For this review, take the finished solid that the model builds, in its own axes (mm). Face numbers are marked on the shaded views. A direction names the side the tool comes from. Round coordinates to 2 decimals unless told otherwise and drop trailing zeros. Loops run counter-clockwise (first coordinate to the right, second up) from the corner with the lowest first, then second, coordinate; pieces in that order, holes last. Notation, with made-up numbers: M 17,22.5 L 49,22.5 A28 ccw 49,43.5 Z; hole C 53.25,26 d6. An arc over 180 degrees is marked long. Write item = value, one per line. Start each with the question number.
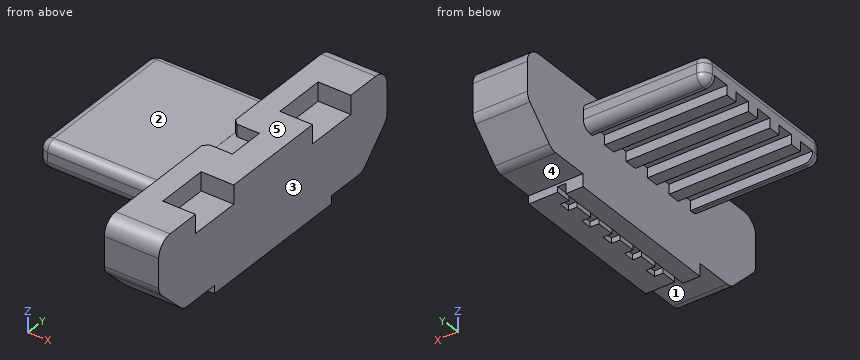
```python
from build123d import *

# Parameters (mm, degrees)
PAD009_DEPTH    = 1.8
PAD008_DEPTH    = 1.2
SKETCH018_W     = 0.214
SKETCH018_H     = 0.247
POCKET007_DEPTH = 0.119
SKETCH019_W     = 0.72
SKETCH019_H     = 1.16
POCKET008_DEPTH = 0.414
POCKET009_DEPTH = 0.27
PAD013_DEPTH    = 2.7
FILLET001_R     = 0.2


with BuildPart() as pad009:
    # Sketch017 → Pad009 (new body, symmetric)
    with BuildSketch(Plane.XZ):
        Polygon((1.529, 0), (1.529, 0.264), (1.708, 0.264), (1.708, 0.145), (2.358, 0.145), (2.358, 0), align=None)
    extrude(amount=PAD009_DEPTH, both=True)


with BuildPart() as part_back:
    # Sketch016 → Pad008 (new body)
    with BuildSketch(Plane(origin=(1.1499999635, -0.0083336435, -0.0078429583), x_dir=(0, 1, 0), z_dir=(1, 0, 0))):
        with BuildLine():
            Line((-3.1093336572, 2.1718425317), (3.1093336572, 2.1718425317))
            ThreePointArc((3.4533336572, 1.8278425317), (3.35257839, 2.0710872645), (3.1093336572, 2.1718425317))
            Line((3.4533336572, 1.8278425317), (3.4533336572, 1.1848425317))
            ThreePointArc((3.3757169542, 0.9974592347), (3.4331617333, 1.0834314222), (3.4533336572, 1.1848425317))
            Line((2.7923538598, 0.4140961402), (3.3757169542, 0.9974592347))
            ThreePointArc((2.588, 0.32945), (2.698595512, 0.3514488151), (2.7923538598, 0.4140961402))
            Line((1.77, 0.32945), (2.588, 0.32945))
            Line((1.77, 0.05045), (1.77, 0.32945))
            Line((1.77, 0.05045), (-1.77, 0.05045))
            Line((-1.77, 0.05045), (-1.77, 0.32945))
            Line((-1.77, 0.32945), (-2.588, 0.32945))
            ThreePointArc((-2.7923538598, 0.4140961402), (-2.698595512, 0.3514488151), (-2.588, 0.32945))
            Line((-3.3757169542, 0.9974592347), (-2.7923538598, 0.4140961402))
            ThreePointArc((-3.4533336572, 1.1848425317), (-3.4331617333, 1.0834314222), (-3.3757169542, 0.9974592347))
            Line((-3.4533336572, 1.8278425317), (-3.4533336572, 1.1848425317))
            ThreePointArc((-3.1093336572, 2.1718425317), (-3.35257839, 2.0710872645), (-3.4533336572, 1.8278425317))
        make_face()
    extrude(amount=PAD008_DEPTH)

    # Cut: cut Pad009
    add(pad009.part, mode=Mode.SUBTRACT)

    # Sketch018 (on Face19 of Cut) → Pocket007 (cut)
    with BuildSketch(Plane(origin=(0, 0, 0.145), x_dir=(1, 0, 0), z_dir=(0, 0, -1))):
        with Locations((1.792, -1.3005)):
            Rectangle(SKETCH018_W, SKETCH018_H)
        with Locations((1.792, -0.6435)):
            Rectangle(SKETCH018_W, SKETCH018_H)
        with Locations((1.792, 0)):
            Rectangle(SKETCH018_W, SKETCH018_H)
        with Locations((1.792, 0.6435)):
            Rectangle(SKETCH018_W, SKETCH018_H)
        with Locations((1.792, 1.3005)):
            Rectangle(SKETCH018_W, SKETCH018_H)
    extrude(amount=-POCKET007_DEPTH, mode=Mode.SUBTRACT)

    # Sketch019 (on Face2 of Pocket007) → Pocket008 (cut)
    with BuildSketch(Plane.XY.offset(2.1639995734)):
        with Locations((1.9899999635, -1.771)):
            Rectangle(SKETCH019_W, SKETCH019_H)
        with Locations((1.9899999635, 1.771)):
            Rectangle(SKETCH019_W, SKETCH019_H)
    extrude(amount=-POCKET008_DEPTH, mode=Mode.SUBTRACT)

    # Sketch020 (on Face2 of Pocket008) → Pocket009 (cut)
    with BuildSketch(Plane.XY.offset(2.1639995734)):
        Polygon((1.249, 0.41), (1.749, 0.41), (1.749, -0.41), (1.249, -0.41), (1.146, -0.513), (1.146, 0.513), align=None)
    extrude(amount=-POCKET009_DEPTH, mode=Mode.SUBTRACT)


with BuildPart() as inner:
    # Sketch029 → Pad013 (new body)
    with BuildSketch(Plane(origin=(-1.5500000108, 1.37e-08, -0.0050004214), x_dir=(0, 1, 0), z_dir=(1, 0, 0))):
        with BuildLine():
            Line((-1.75, 1.6999999949), (-1.75, 1.5000000051))
            ThreePointArc((-1.75, 1.5000000051), (-1.6914213581, 1.3585786456), (-1.55, 1.3))
            Line((-1.55, 1.3), (-1.486, 1.3))
            Line((-1.486, 1.3), (-1.486, 1.514))
            Line((-1.486, 1.514), (-1.115, 1.514))
            Line((-1.115, 1.514), (-1.115, 1.3))
            Line((-1.115, 1.3), (-0.837, 1.3))
            Line((-0.837, 1.3), (-0.837, 1.514))
            Line((-0.837, 1.514), (-0.466, 1.514))
            Line((-0.466, 1.514), (-0.466, 1.3))
            Line((-0.466, 1.3), (-0.188, 1.3))
            Line((-0.188, 1.3), (-0.188, 1.514))
            Line((-0.188, 1.514), (0.183, 1.514))
            Line((0.183, 1.514), (0.183, 1.3))
            Line((0.183, 1.3), (0.461, 1.3))
            Line((0.461, 1.3), (0.461, 1.514))
            Line((0.461, 1.514), (0.832, 1.514))
            Line((0.832, 1.514), (0.832, 1.3))
            Line((0.832, 1.3), (1.11, 1.3))
            Line((1.11, 1.3), (1.11, 1.514))
            Line((1.11, 1.514), (1.481, 1.514))
            Line((1.481, 1.514), (1.481, 1.3))
            Line((1.481, 1.3), (1.55, 1.3))
            ThreePointArc((1.55, 1.3), (1.6914213581, 1.3585786456), (1.75, 1.5000000051))
            Line((1.75, 1.6999999949), (1.75, 1.5000000051))
            ThreePointArc((1.75, 1.6999999949), (1.6914213581, 1.8414213544), (1.55, 1.9))
            Line((-1.55, 1.9), (1.55, 1.9))
            ThreePointArc((-1.55, 1.9), (-1.6914213581, 1.8414213544), (-1.75, 1.6999999949))
        make_face()
    extrude(amount=PAD013_DEPTH)

    # Fillet001
    fillet001_edges = [inner.edges().sort_by_distance(p)[0] for p in [
        (-1.55, -1.75, 1.595),
        (-1.55, -1.691421, 1.353578),
        (-1.55, 1.691421, 1.353578),
        (-1.55, 1.75, 1.595),
        (-1.55, 1.691421, 1.836421),
        (-1.55, 0, 1.895),
        (-1.55, -1.691421, 1.836421),
    ]]
    fillet(fillet001_edges, radius=FILLET001_R)

    # Fusion002: union Part-back
    add(part_back.part)


solid = inner.part
```
(1) Wall thickness on L1, parallel to Y at x = 2.15, z = 1.8 (3 decimals); L2, parallel to X at y = 0.5, z = 0.8; L3, parallel to Z at x = 1.75, y = -2.5: over which ranges is each line inside the solid? List them lowest first.
(2) Add section C-C on x = 0.4. Write out the cut boundary in (y, z) (3 decimals), and give its area (3 significant figures).
(3) Add section A-A on x = 2.15. Write out the cut boundary in (y, z) (3 decimals), and give its area (3 significant figures).
(4) Tool access review of the marked faces 1, 2, 3, 4 and 5: name each direction out of +Z, -Z, +X, -X, +Y, -Y from which nothing blocks a thin tool from reaching the whole face with its end or side.
(5) Add section B-B on y = 2. Write out the cut boundary in (x, z), and give its area (3 significant figures).
(6) For pin 1 Ø0.7 at (x, y) = (2, -2) entering from -Z (3 decimals), flat-tipped, find the tip position at first contact; note if it passes through.
Answer sheet:
q1.L1 = -3.462 to -2.351, -1.191 to 1.191, 2.351 to 3.445
q1.L2 = 1.15 to 2.35
q1.L3 = 0.32 to 2.16
q2.outline = M -1.75,1.495 A0.2 ccw -1.55,1.295 L -1.486,1.295 L -1.486,1.509 L -1.115,1.509 L -1.115,1.295 L -0.837,1.295 L -0.837,1.509 L -0.466,1.509 L -0.466,1.295 L -0.188,1.295 L -0.188,1.509 L 0.183,1.509 L 0.183,1.295 L 0.461,1.295 L 0.461,1.509 L 0.832,1.509 L 0.832,1.295 L 1.11,1.295 L 1.11,1.509 L 1.481,1.509 L 1.481,1.295 L 1.55,1.295 A0.2 ccw 1.75,1.495 L 1.75,1.695 A0.2 ccw 1.55,1.895 L -1.55,1.895 A0.2 ccw -1.75,1.695 Z
q2.area = 1.67 mm²
q3.outline = M -3.462,1.177 A0.265 ccw -3.384,0.99 L -2.801,0.406 A0.289 ccw -2.596,0.322 L -1.778,0.322 L -1.778,0.145 L 1.762,0.145 L 1.762,0.322 L 2.58,0.322 A0.289 ccw 2.784,0.406 L 3.367,0.99 A0.265 ccw 3.445,1.177 L 3.445,1.82 A0.344 ccw 3.101,2.164 L 2.351,2.164 L 2.351,1.75 L 1.191,1.75 L 1.191,2.164 L -1.191,2.164 L -1.191,1.75 L -2.351,1.75 L -2.351,2.164 L -3.118,2.164 A0.344 ccw -3.462,1.82 Z
q3.area = 11.8 mm²
q4.face_1 = -Z, +X, -X, -Y
q4.face_2 = +Z, -X, +Y, -Y
q4.face_3 = +Z, -Z, +X, +Y, -Y
q4.face_4 = -Z, +X, -X, +Y
q4.face_5 = +Z, +X, -X, +Y, -Y
q5.outline = M 1.15,0.32 L 2.35,0.32 L 2.35,1.75 L 1.63,1.75 L 1.63,2.16 L 1.15,2.16 Z
q5.area = 1.91 mm²
q6.pin_1 = 0.145
